from build123d import *

# Parameters (mm, degrees)
F0_W      = 50
F0_H      = 60
F1_DEPTH  = 5
F4_START  = 2
F3_W      = 58
F3_H      = 60
F4_DEPTH  = 3
F2_W      = 45.5
F2_H      = 45.5
F5_DEPTH  = 3
F7_START  = 1.5
F6_W      = 20
F6_H      = 30
F7_DEPTH  = 1.5
F8_W      = 2
F8_H      = 56
F9_DEPTH  = 25
F10_R     = 2
F11_W     = 5
F11_H     = 1.5
F12_DEPTH = 2
F13_SIZE  = 1.5
F15_START = 3
F14_W     = 20
F14_H     = 3
F15_DEPTH = 2


with BuildPart() as f1:
    # F0 (on Top) → F1 (new body)
    with BuildSketch(Plane.XY):
        Rectangle(F0_W, F0_H)
    extrude(amount=F1_DEPTH)

    # F3 (on Top) → F4 (join)
    with BuildSketch(Plane.XY.offset(F4_START)):
        Rectangle(F3_W, F3_H)
    extrude(amount=F4_DEPTH)

    # F2 (on Top) → F5 (cut)
    with BuildSketch(Plane.XY):
        Rectangle(F2_W, F2_H)
    extrude(amount=F5_DEPTH, mode=Mode.SUBTRACT)

    # F6 (on Top) → F7 (cut)
    with BuildSketch(Plane.XY.offset(F7_START)):
        with Locations((0, -15)):
            Rectangle(F6_W, F6_H)
    extrude(amount=F7_DEPTH, mode=Mode.SUBTRACT)

    # F8 (on Top) → F9 (cut)
    with BuildSketch(Plane.XY):
        with Locations((-26, 0)):
            Rectangle(F8_W, F8_H)
        with Locations((26, 0)):
            Rectangle(F8_W, F8_H)
    extrude(amount=F9_DEPTH, mode=Mode.SUBTRACT)

    # F10
    f10_edges = [f1.edges().sort_by_distance(p)[0] for p in [
        (29, -30, 3.5),
        (-29, -30, 3.5),
        (-29, 30, 3.5),
        (29, 30, 3.5),
    ]]
    fillet(f10_edges, radius=F10_R)

    # F11 (on Top) → F12 (join)
    with BuildSketch(Plane.XY):
        with Locations((-14.75, -30.75)):
            Rectangle(F11_W, F11_H)
        with Locations((14.75, -30.75)):
            Rectangle(F11_W, F11_H)
        with Locations((14.75, 30.75)):
            Rectangle(F11_W, F11_H)
        with Locations((-14.75, 30.75)):
            Rectangle(F11_W, F11_H)
    extrude(amount=F12_DEPTH)

    # F13
    f13_edges = [f1.edges().sort_by_distance(p)[0] for p in [
        (-14.75, -31.5, 0),
        (14.75, -31.5, 0),
        (14.75, 31.5, 0),
        (-14.75, 31.5, 0),
    ]]
    chamfer(f13_edges, length=F13_SIZE)

    # F14 (on Top) → F15 (cut)
    with BuildSketch(Plane.XY.offset(F15_START)):
        with Locations((0, -28.5)):
            Rectangle(F14_W, F14_H)
    extrude(amount=F15_DEPTH, mode=Mode.SUBTRACT)


solid = f1.part
Check sheet for the modelled part. Datum: model origin and axes. Units: mm. A direction names the side the tool comes from. Round coordinates to 2 decimals unless told otherwise and drop trailing zeros. Order: outer loops, then holes, each group sorted by start corner. A loop starts at its lowest first (then second) coordinate and runs counter-clockwise, first axis right, second up.
(1) Cross-section at D-D, the plane y = -7. Enter the section's corners in (x, z).
(2) Cross-section at A-A, the plane y = -24. Enter the section's corners in (x, z).
(3) Access from +Z, -Z, +X, -X, +Y, -Y to the whole of each face (thin tool, end or side, straight path). Record for faces 1 (the flat face through (0, -27, 4)), 2 (the flat face through (-15, -31, 2)), 3 (the flat face through (0, -26, 1.5)).
(4) Cross-section at C-C, the plane z = 4.15. Enter the section's corners in (x, y), and give its area (3 significant figures).
(5) Scan lines: probe 1 along X at (y, z) = (-23, 3.6); probe 2 along X at (y, z) = (22.5, 2.85); probe 3 along Y at (x, z) = (-21.5, 2.8). Record each from-to range of solid material in increasing order.
(6) Cross-section at B-B, the plane x = -1.5. Enter the section's corners in (y, z).
(7) Draft check along X on faces 4 (the flat face through (0, 22.75, 1)), 5 (the flat face through (-15, 31, 1)), 6 (the cylindrical face through (-28.43, 29.4, 3.52)). Enter one of: pulls with the +X half, pulls with the -X half, needs draft (parallel to the pull), parting line crosses it, or undercut.
(8) Go/stop test with flat-tipped pins: P1, Ø2.5, axis at x = 4, z = 2, coming from the +Y side; P2, Ø1.2, axis at y = -30.5, z = 1.5, coming from the -X side; P3, Ø8, axis at x = 4, y = -7, coming from the -Z side. Record where each tip stops, or that it passes through.
Check sheet entries:
1. outline: (-29, 2) - (-27, 2) - (-27, 5) - (-29, 5) - close; (-25, 0) - (-22.75, 0) - (-22.75, 3) - (22.75, 3) - (22.75, 0) - (25, 0) - (25, 5) - (-25, 5) - close; (27, 2) - (29, 2) - (29, 5) - (27, 5) - close
2. outline: (-29, 2) - (-27, 2) - (-27, 5) - (-29, 5) - close; (-25, 0) - (25, 0) - (25, 5) - (-25, 5) - close; (27, 2) - (29, 2) - (29, 5) - (27, 5) - close; hole (-10, 1.5) - (10, 1.5) - (10, 3) - (-10, 3) - close
3. face 1: +Z, -Y
3. face 2: +Z, +X, -X, -Y
3. face 3: -Y
4. outline: (-29, -28) arc R2 ccw to (-27, -30) - (-10, -30) - (-10, -27) - (10, -27) - (10, -30) - (27, -30) arc R2 ccw to (29, -28) - (29, 28) arc R2 ccw to (27, 30) - (-27, 30) arc R2 ccw to (-29, 28) - close; hole (-27, -28) - (-25, -28) - (-25, 28) - (-27, 28) - close; hole (25, -28) - (27, -28) - (27, 28) - (25, 28) - close
4. area: 3,190 mm2
5. probe 1: x = -29 to -27, -25 to 25, 27 to 29
5. probe 2: x = -29 to -27, -25 to -22.75, 22.75 to 25, 27 to 29
5. probe 3: y = -30 to -22.75, 22.75 to 30
6. outline: (-30, 0) - (-22.75, 0) - (-22.75, 1.5) - (-30, 1.5) - close; (-27, 3) - (22.75, 3) - (22.75, 0) - (30, 0) - (30, 5) - (-27, 5) - close
7. face 4: undercut
7. face 5: needs draft
7. face 6: pulls with the -X half
8. P1: stops at y = 30
8. P2: stops at x = -25
8. P3: stops at z = 3
